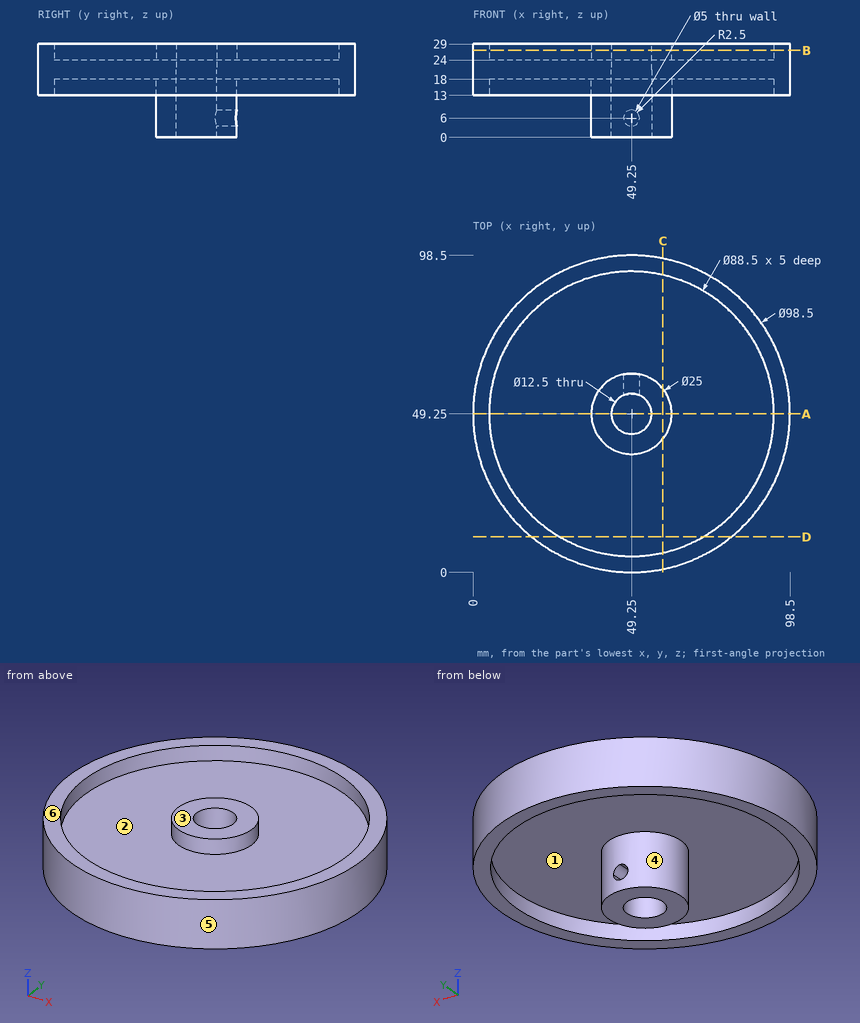
The figure shows three views and two pictorial views of one solid part (mm, origin at its lowest corner). Answer the questions. A direction names the side the tool comes from. Round coordinates to 2 decimals unless told otherwise and drop trailing zeros. Order: outer loops, then holes, each group sorted by start corner. A loop starts at its lowest first (then second) coordinate and runs counter-clockwise, first axis right, second up.
Q1. A cutting plane is placed at A-A, the plane y = 49.25. Determine the outline of the cut face in (x, z).
Solution:
outline: (0, 13) - (5, 13) - (5, 18) - (36.75, 18) - (36.75, 0) - (43, 0) - (43, 29) - (36.75, 29) - (36.75, 24) - (5, 24) - (5, 29) - (0, 29) - close; (55.5, 0) - (61.75, 0) - (61.75, 18) - (93.5, 18) - (93.5, 13) - (98.5, 13) - (98.5, 29) - (93.5, 29) - (93.5, 24) - (61.75, 24) - (61.75, 29) - (55.5, 29) - close
Q2. Find the intervals of material crossed by line 1 along Y through (x, z) = (49.25, 27.3); line 2 along Z through (x, y) = (49, 57); line 3 along Z through (x, y) = (78.5, 87.5), in increasing order.
Solution:
line 1: y = 0 to 5, 36.75 to 43, 55.5 to 61.75, 93.5 to 98.5
line 2: z = 0 to 3.51, 8.49 to 29
line 3: z = 13 to 29
Q3. A cutting plane is placed at D-D, the plane y = 11. Determine the outline of the cut face in (x, z).
Solution:
outline: (18.23, 13) - (27, 13) - (27, 18) - (71.5, 18) - (71.5, 13) - (80.27, 13) - (80.27, 29) - (71.5, 29) - (71.5, 24) - (27, 24) - (27, 29) - (18.23, 29) - close
Q4. A cutting plane is placed at B-B, the plane z = 27. Determine the outline of the cut face in (x, y).
Solution:
outline: circle Ø98.5 at (49.25, 49.25); circle Ø25 at (49.25, 49.25); hole circle Ø88.5 at (49.25, 49.25); hole circle Ø12.5 at (49.25, 49.25)
Q5. The mould has two halves that part along X. Classify the marked faces 4, 5 and 6: pulls with the +X half, pulls with the -X half, needs draft (parallel to the pull), parting line crosses it, or undercut.
Solution:
face 4: undercut
face 5: parting line crosses it
face 6: needs draft
Q6. Given pin 1 Ø3 at (x, y) = (18, 69.5) entering from -Z; pin 2 Ø3 at (y, z) = (62, 22) entering from -X; pin 3 Ø5 at (x, z) = (70, 25) entering from +Y; pin 4 Ø11 at (x, y) = (49.25, 49.25) entering from -Z, each flat-ended and moving along its own axis, determine where each tip first touches the part or whether it passes through.
Solution:
pin 1: stops at z = 18
pin 2: stops at x = 1.3
pin 3: stops at y = 94.99
pin 4: passes through
Q7. A tool of negligible diameter and unlimited length cuts with its end or side. For the marked faces 1, 2 and 3, from which of +Z, -Z, +X, -X, +Y, -Y can it reach the whole face along a straight path? Write none if from no direction.
Solution:
face 1: -Z
face 2: +Z
face 3: +Z, +X, -X, +Y, -Y
Q8. A cutting plane is placed at C-C, the plane x = 59. Determine the outline of the cut face in (y, z), then the cut area to 3 significant figures.
Solution:
outline: (0.97, 13) - (6.09, 13) - (6.09, 18) - (41.43, 18) - (41.43, 0) - (57.07, 0) - (57.07, 18) - (92.41, 18) - (92.41, 13) - (97.53, 13) - (97.53, 29) - (92.41, 29) - (92.41, 24) - (57.07, 24) - (57.07, 29) - (41.43, 29) - (41.43, 24) - (6.09, 24) - (6.09, 29) - (0.97, 29) - close
area: 1,040 mm2
